Could you check a few things on this model? Use its own coordinates, in mm. Coordinates: 2 decimals unless noted, no trailing zeros. Write each loop counter-clockwise with the first axis right and the second up, starting at its lowest first coordinate (ties: lowest second). Pieces come first, ordered by that corner, then holes. Notation, with made-up numbers: M 78.25,28 L 119.25,28 A16 ccw 119.25,39 Z; hole C 62.25,62 d4. An arc over 180 degrees is marked long. Answer as CSV lines item,"result". Start each with the question number.
Item 1: Suppose I cut it at B-B, the plane z = 0.55. State how many separate pieces and enclosed holes the cut face has, and give its area (3 significant figures).
Item 2: Suppose I cut it at A-A, the plane x = 60. Write out the boundary of the cut face in (y, z), and give its area (3 significant figures).
Item 3: If I drill on line 1 along X through (y, z) = (90, 1); line 2 along Y through (x, z) = (50.5, 0.6); line 3 along X through (y, z) = (13, 2.3), over which ranges is the centre line in solid material (lowest first)? Write a range as [from, to].
Item 4: I'm going to push a flat-ended pin straight in: P1, Ø1.5, axis at y = 128.5, z = 1.5, coming from the +X side. Where does the tip first touch, or does it pass through?
```python
from build123d import *

# Parameters (mm, degrees)
SKETCH1_W           = 125
SKETCH1_H           = 150
BOSS_EXTRUDE1_DEPTH = 3
SKETCH6_R           = 1.5
CUT_EXTRUDE5_DEPTH  = 4
CUT_EXTRUDE6_DEPTH  = 4
SKETCH8_R           = 1.5
CUT_EXTRUDE7_DEPTH  = 4.0000001
FILLET1_R           = 10
SKETCH10_W          = 58.197172172
SKETCH10_H          = 21.139257973
CUT_EXTRUDE8_DEPTH  = 4.0000001
SKETCH11_W          = 3
SKETCH11_H          = 10
CUT_EXTRUDE9_DEPTH  = 4.0000001


with BuildPart() as part:
    # Sketch1 → Boss-Extrude1 (new body)
    with BuildSketch(Plane.XY):
        with Locations((62.5, 75)):
            Rectangle(SKETCH1_W, SKETCH1_H)
    extrude(amount=BOSS_EXTRUDE1_DEPTH)

    # Sketch6 → Cut-Extrude5 (cut, through all)
    with BuildSketch(Plane(origin=(0, 0, 0), x_dir=(-1, 0, 0), z_dir=(0, 0, -1))):
        with Locations((-15.5, 135.678181118)):
            Circle(SKETCH6_R)
        with Locations((-109.5, 135.678181118)):
            Circle(SKETCH6_R)
    extrude(amount=-CUT_EXTRUDE5_DEPTH, mode=Mode.SUBTRACT)

    # Sketch7 → Cut-Extrude6 (cut, through all)
    with BuildSketch(Plane.XY.offset(3)):
        with BuildLine():
            Line((18.83856041, 150), (0, 150))
            Line((0, 150), (0, 121.303805561))
            add(Edge.make_bspline(
                [(0, 121.303805561), (5.130729703, 138.554109372), (8.057120528, 143.174726465), (13.293819899, 147.487302418), (18.83856041, 150)],
                knots=[0, 0, 0, 0, 0, 1, 1, 1, 1, 1], degree=4))
        make_face()
        with BuildLine():
            Line((125, 150), (125, 121.303805561))
            add(Edge.make_bspline(
                [(125, 121.303805561), (119.869270297, 138.554109372), (116.942879472, 143.174726465), (111.706180101, 147.487302418), (106.16143959, 150)],
                knots=[0, 0, 0, 0, 0, 1, 1, 1, 1, 1], degree=4))
            Line((106.16143959, 150), (125, 150))
        make_face()
    extrude(amount=-CUT_EXTRUDE6_DEPTH, mode=Mode.SUBTRACT)

    # Sketch8 → Cut-Extrude7 (cut, through all)
    with BuildSketch(Plane.XY.offset(3)):
        with Locations((14.8, 12)):
            Circle(SKETCH8_R)
        with Locations((110.2, 12)):
            Circle(SKETCH8_R)
        with Locations((14.8, 90)):
            Circle(SKETCH8_R)
        with Locations((110.2, 90)):
            Circle(SKETCH8_R)
    extrude(amount=-CUT_EXTRUDE7_DEPTH, mode=Mode.SUBTRACT)

    # Fillet1
    fillet1_edges = [part.edges().sort_by_distance(p)[0] for p in [
        (125, 0, 1.5),
        (0, 0, 1.5),
    ]]
    fillet(fillet1_edges, radius=FILLET1_R)

    # Sketch10 → Cut-Extrude8 (cut, through all)
    with BuildSketch(Plane.XY.offset(3)):
        with Locations((62.5, 80.404070369)):
            Rectangle(SKETCH10_W, SKETCH10_H)
    extrude(amount=-CUT_EXTRUDE8_DEPTH, mode=Mode.SUBTRACT)

    # Sketch11 → Cut-Extrude9 (cut, through all)
    with BuildSketch(Plane.XY.offset(3)):
        with Locations((72, 130)):
            Rectangle(SKETCH11_W, SKETCH11_H)
        with Locations((53, 130)):
            Rectangle(SKETCH11_W, SKETCH11_H)
    extrude(amount=-CUT_EXTRUDE9_DEPTH, mode=Mode.SUBTRACT)


solid = part.part
```
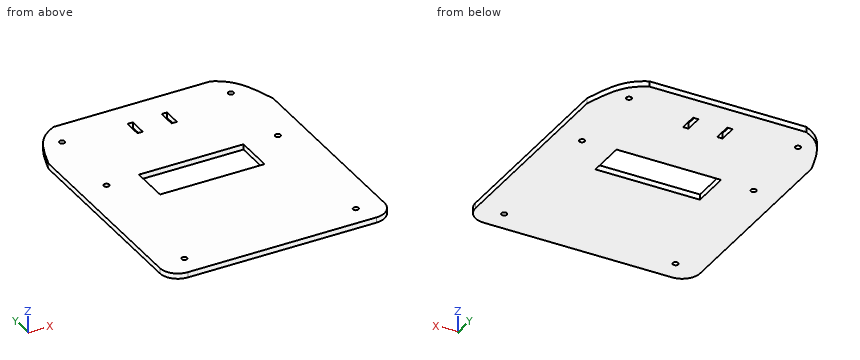
Ans:
1,separate pieces,"1"
1,enclosed holes,"9"
1,area,"17,000 mm^2"
2,outline,"M 0,0 L 69.83,0 L 69.83,3 L 0,3 Z; M 90.97,0 L 150,0 L 150,3 L 90.97,3 Z"
2,area,"387 mm^2"
3,line 1,"x = [0, 13.3], [16.3, 33.4], [91.6, 108.7], [111.7, 125]"
3,line 2,"y = [0, 69.83], [90.97, 150]"
3,line 3,"x = [0, 13.68], [15.92, 109.08], [111.32, 125]"
4,P1,"stops at x = 122.98"
